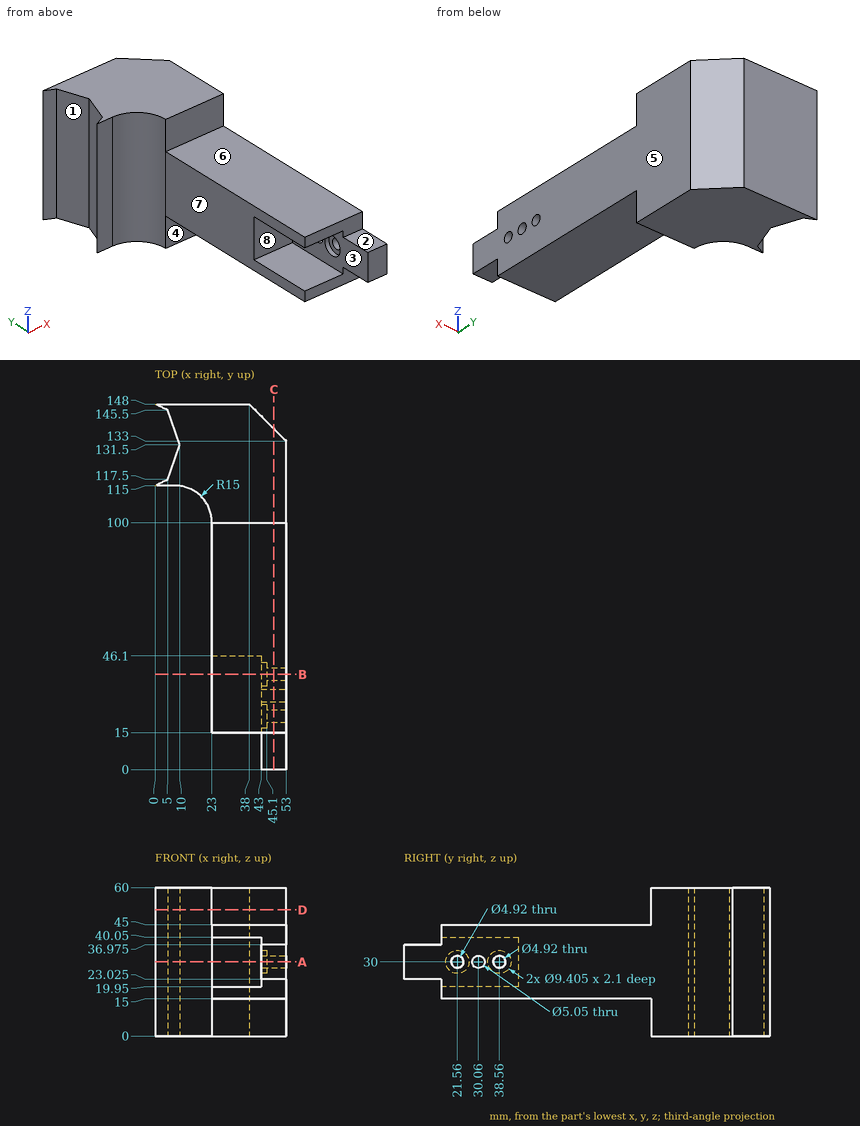
Verification items for this drawing (mm, ordinates from the low corner). A direction names the side the tool comes from. Round coordinates to 2 decimals unless told otherwise and drop trailing zeros. Order: outer loops, then holes, each group sorted by start corner. A loop starts at its lowest first (then second) coordinate and runs counter-clockwise, first axis right, second up. Notation, with made-up numbers: M -3,44 L 43,44 A8 cw 43,49 Z; hole C -20,-20.5 d8. An arc over 180 degrees is marked long. Answer in a Markdown table with one row per item. Add a question column.
Item 1: Sectioned sample at C-C, the plane x = 48. Enter the section's corners in (y, z) (3 decimals).
Item 2: Set-up check for the marked faces 4, 5, 6, 7 and 8: record each of +Z, -Z, +X, -X, +Y, -Y from which the full face is reachable in a straight line by a thin tool's end or side.
Item 3: Depth check by flat-ended pin: pin 1 Ø6 at (y, z) = (26, 37.5) entering from -X; pin 2 Ø4.5 at (y, z) = (22.5, 29) entering from -X; pin 3 Ø6 at (x, y) = (32, 34.5) entering from +Z. Enter the tip coordinate at first touch or a pass-through.
Item 4: Sectioned sample at D-D, the plane z = 51. Enter the section's corners in (x, y), plus the area to 3 significant figures.
Item 5: Sectioned sample at B-B, the plane y = 38.56. Enter the section's corners in (x, z).
Item 6: Material ranges on L1, parallel to Z at x = 49.75, y = 38.56; L2, parallel to Y at x = 44.2, z = 30 (1 decimal); L3, parallel to Y at x = 48, z = 30 (3 decimals), recorded low to high. Write a range as [from, to].
Item 7: Draft check along Z on the marked faces 1, 2 and 3. Enter one of: released by +Z, released by -Z, zero draft, split by the parting line, or undercut.
Item 8: Sectioned sample at A-A, the plane z = 30. State how many separate pieces and enclosed holes the cut face has, plus the area to 3 significant figures.
Filled in:
| question | item | result |
|---|---|---|
| 1 | outline | M 0,23.025 L 15,23.025 L 15,15 L 100,15 L 100,0 L 138,0 L 138,60 L 100,60 L 100,45 L 15,45 L 15,36.975 L 0,36.975 Z; hole C 21.56,30 d4.92; hole C 30.06,30 d5.05; hole C 38.56,30 d4.92 |
| 2 | face 4 | -Z, +X, -X, -Y |
| 2 | face 5 | +Z, -Z, +X, +Y, -Y |
| 2 | face 6 | +Z, +X, -X, -Y |
| 2 | face 7 | +Z, -Z, -X, -Y |
| 2 | face 8 | -X, -Y |
| 3 | pin 1 | stops at x = 23 |
| 3 | pin 2 | stops at x = 45.1 |
| 3 | pin 3 | stops at z = 45 |
| 4 | outline | M 0,115 L 8,115 A15 cw 23,100 L 53,100 L 53,133 L 38,148 L 0,148 L 5,145.5 L 10,131.5 L 5,117.5 Z |
| 4 | area | 1,910 mm² |
| 5 | outline | M 23,15 L 53,15 L 53,27.54 L 45.1,27.54 L 45.1,25.3 L 43,25.3 L 43,19.95 L 23,19.95 Z; M 23,40.05 L 43,40.05 L 43,34.7 L 45.1,34.7 L 45.1,32.46 L 53,32.46 L 53,45 L 23,45 Z |
| 6 | L1 | z = [15, 27.54], [32.46, 45] |
| 6 | L2 | y = [0, 16.9], [26.3, 27.5], [32.6, 33.9], [43.3, 141.8] |
| 6 | L3 | y = [0, 19.1], [24.02, 27.535], [32.585, 36.1], [41.02, 138] |
| 7 | face 1 | zero draft |
| 7 | face 2 | released by +Z |
| 7 | face 3 | undercut |
| 8 | separate pieces | 4 |
| 8 | enclosed holes | 0 |
| 8 | area | 3,820 mm² |
